Input: part model. Units: mm. Frame: model coordinates. A direction names the side the tool comes from. Give positions to 0.01 mm unless a question says otherwise; leave off trailing zeros. Loops run counter-clockwise (first coordinate to the right, second up) from the corner with the lowest first, then second, coordinate; pieces in that order, holes last. Notation, with made-up numbers: M 47.5,17.5 L 101.5,17.5 A29 ccw 101.5,45.5 Z; hole C 41.25,4.5 d8. An arc over 180 degrees is marked long. Use CSV: the item, a comma, the result in double quotes. Start each with the question number.
Q1. Pin query (flat end, axial travel): pin 1 (3.5 mm diameter, centred on x = 36, z = -3.5, fed in from +Y); pin 2 (2 mm diameter, centred on x = -11, z = -3.5, fed in from +Y); pin 3 (8 mm diameter, centred on x = 13.5, y = -80.5, fed in from -Z). Return the tip coordinate at first contact, or that it passes through.
Q2. Material intervals for line 1 along Y through (x, z) = (36.5, -1.75); line 2 along Y through (x, z) = (6.5, -5.5); line 3 along Z through (x, y) = (-1, -86.5), sorted ascending.
Q3. Section D-D, the plane y = -17. Output: boundary loops of the cut face in (x, z), plus the area to 3 significant figures.
Q4. Pull-direction query (Y, two-part tool) for faces 5 (the flat face through (-22, -88.099, -3)), 6 (the flat face through (8, -19, -5)), 7 (the cylindrical face through (-38.079, -21.806, -2.465)); classes: released by +Y, released by -Y, zero draft, split by the parting line, or undercut.
Q5. Reachability of faces 1 (the flat face through (38, -18.099, -3)), 2 (the flat face through (-36.523, -52.791, -2.535)), 3 (the flat face through (7.92, -93.59, -6.17)), 4 (the flat face through (-22, -18.099, -3)) from +Z, -Z, +X, -X, +Y, -Y: full face, straight path, thin tool, end or side. Return the list, or none.
from build123d import *

# Parameters (mm, degrees)
BOSS_EXTRUDE1_DEPTH       = 5
CHAMFER1_SIZE             = 5
BOSS_EXTRUDE2_DEPTH       = 8
CHAMFER2_SIZE2            = 5
CHAMFER2_SIZE             = 8.660254038
CHAMFER2_OF_MIRROR1_SIZE2 = 5
CHAMFER2_OF_MIRROR1_SIZE  = 8.660254038


# Some blends are built 0.0001 mm under size
with BuildPart() as part:
    # Sketch1 → Boss-Extrude1 (new body)
    # profile 1 of 2: a face of its own
    with BuildSketch(Plane.XY):
        with BuildLine():
            Line((-41.988438617, -31.098685124), (-41.988438617, -75.098685124))
            ThreePointArc((-41.988438617, -75.098685124), (-38.180826772, -84.291073279), (-28.988438617, -88.098685124))
            Line((-28.988438617, -88.098685124), (45.011561383, -88.098685124))
            ThreePointArc((45.011561383, -88.098685124), (54.203949538, -84.291073279), (58.011561383, -75.098685124))
            Line((58.011561383, -75.098685124), (58.011561383, -31.098685124))
            ThreePointArc((58.011561383, -31.098685124), (54.203949538, -21.906296968), (45.011561383, -18.098685124))
            Line((45.011561383, -18.098685124), (-28.988438617, -18.098685124))
            ThreePointArc((-28.988438617, -18.098685124), (-38.180826772, -21.906296968), (-41.988438617, -31.098685124))
        make_face()
        with BuildLine():
            ThreePointArc((-38.988438617, -75.098685124), (-36.059506429, -82.169752935), (-28.988438617, -85.098685124))
            Line((-28.988438617, -85.098685124), (45.011561383, -85.098685124))
            ThreePointArc((45.011561383, -85.098685124), (52.082629195, -82.169752935), (55.011561383, -75.098685124))
            Line((55.011561383, -75.098685124), (55.011561383, -31.098685124))
            ThreePointArc((55.011561383, -31.098685124), (52.082629195, -24.027617312), (45.011561383, -21.098685124))
            Line((45.011561383, -21.098685124), (-28.988438617, -21.098685124))
            ThreePointArc((-28.988438617, -21.098685124), (-36.059506429, -24.027617312), (-38.988438617, -31.098685124))
            Line((-38.988438617, -31.098685124), (-38.988438617, -75.098685124))
        make_face(mode=Mode.SUBTRACT)
    # profile 2 of 2: a face of its own
    with BuildSketch(Plane.XY):
        with BuildLine():
            Line((-38.988438617, -31.098685124), (-38.988438617, -75.098685124))
            ThreePointArc((-38.988438617, -75.098685124), (-36.059506429, -82.169752935), (-28.988438617, -85.098685124))
            Line((-28.988438617, -85.098685124), (45.011561383, -85.098685124))
            ThreePointArc((45.011561383, -85.098685124), (52.082629195, -82.169752935), (55.011561383, -75.098685124))
            Line((55.011561383, -75.098685124), (55.011561383, -31.098685124))
            ThreePointArc((55.011561383, -31.098685124), (52.082629195, -24.027617312), (45.011561383, -21.098685124))
            Line((45.011561383, -21.098685124), (-28.988438617, -21.098685124))
            ThreePointArc((-28.988438617, -21.098685124), (-36.059506429, -24.027617312), (-38.988438617, -31.098685124))
        make_face()
        with BuildLine():
            ThreePointArc((-33.988438617, -75.098685124), (-32.523972523, -78.63421903), (-28.988438617, -80.098685124))
            Line((-28.988438617, -80.098685124), (45.011561383, -80.098685124))
            ThreePointArc((45.011561383, -80.098685124), (48.547095289, -78.63421903), (50.011561383, -75.098685124))
            Line((50.011561383, -75.098685124), (50.011561383, -31.098685124))
            ThreePointArc((50.011561383, -31.098685124), (48.547095289, -27.563151218), (45.011561383, -26.098685124))
            Line((45.011561383, -26.098685124), (-28.988438617, -26.098685124))
            ThreePointArc((-28.988438617, -26.098685124), (-32.523972523, -27.563151218), (-33.988438617, -31.098685124))
            Line((-33.988438617, -31.098685124), (-33.988438617, -75.098685124))
        make_face(mode=Mode.SUBTRACT)
    extrude(amount=-BOSS_EXTRUDE1_DEPTH)

    # Chamfer1
    chamfer1_edges = [part.edges().sort_by_distance(p)[0] for p in [
        (8.011561383, -80.098685124, -5),
        (48.547095289, -78.63421903, -5),
        (-32.523972523, -78.63421903, -5),
        (50.011561383, -53.098685124, -5),
        (-33.988438617, -53.098685124, -5),
        (48.547095289, -27.563151218, -5),
        (-32.523972523, -27.563151218, -5),
        (8.011561383, -26.098685124, -5),
    ]]
    chamfer(chamfer1_edges, length=CHAMFER1_SIZE - 0.0001)  # a hair under: the kernel refuses the full size

    # Sketch2 → Boss-Extrude2 (add)
    with BuildSketch(Plane.XY):
        Polygon((-15.345428916, -18.098685124), (-7.774377041, -10.527633249), (23.073373404, -10.527633249), (30.644425279, -18.098685124), align=None)
    boss_extrude2 = extrude(amount=-BOSS_EXTRUDE2_DEPTH)

    # Chamfer2
    chamfer2_edges = [part.edges().sort_by_distance(p)[0] for p in [
        (7.649498182, -10.527633249, 0),
    ]]
    chamfer2_side = [part.faces().sort_by_distance(p)[0] for p in [
        (7.649498182, -10.627633249, 0),
    ]]
    chamfer(chamfer2_edges, length=CHAMFER2_SIZE, length2=CHAMFER2_SIZE2, reference=chamfer2_side[0])
    # the kernel refuses this chamfer: 8.660254038, 5 mm, written as the material it takes off along each edge
    with BuildSketch(Plane(origin=(53.049245132, -18.098685124, -8), x_dir=(0, -0.05789386240267115, 0.9983227437537926), z_dir=(-1, 0, 0))) as chamfer2_2_piece_1_section:
        with BuildLine():
            Line((5.181896449, 0), (-0.691658286, 8.935197885))
            Line((-0.691658286, 8.935197885), (-0.864572857, 8.925170374))
            ThreePointArc((-0.864572857, 8.925170374), (-0.432286429, 4.462585187), (-0.172914571, -0.010027511))
            Line((-0.172914571, -0.010027511), (0.010027511, -0.172914571))
            ThreePointArc((0.010027511, -0.172914571), (2.592291656, -0.02316616), (5.19192396, -0.172914571))
            Line((5.19192396, -0.172914571), (5.181896449, 0))
        make_face()
    chamfer2_2_piece_1 = extrude(amount=90.7994939, mode=Mode.PRIVATE)
    chamfer2_2_piece_1 = split(chamfer2_2_piece_1, bisect_by=Plane(origin=(7.649498182, -14.797310686, -5), z_dir=(0, 0, -1)), keep=Keep.TOP, mode=Mode.PRIVATE)
    add(chamfer2_2_piece_1, mode=Mode.SUBTRACT)

    # Mirror1: Boss-Extrude2 across plane
    add(boss_extrude2.mirror(Plane.ZX.offset(-53.098685124)))

    # Chamfer2 of Mirror1
    chamfer2_of_mirror1_edges = [part.edges().sort_by_distance(p)[0] for p in [
        (7.649498182, -95.669736998, 0),
    ]]
    chamfer2_of_mirror1_side = [part.faces().sort_by_distance(p)[0] for p in [
        (7.649498182, -95.569736998, 0),
    ]]
    chamfer(chamfer2_of_mirror1_edges, length=CHAMFER2_OF_MIRROR1_SIZE, length2=CHAMFER2_OF_MIRROR1_SIZE2, reference=chamfer2_of_mirror1_side[0])
    # the kernel refuses this chamfer: 8.660254038, 5 mm, written as the material it takes off along each edge
    with BuildSketch(Plane(origin=(53.049245132, -88.098685124, -8), x_dir=(0, 0.057893862402670464, 0.9983227437537926), z_dir=(-1, 0, 0))) as chamfer2_of_mirror1_2_piece_1_section:
        with BuildLine():
            Line((5.181896449, 0), (-0.691658286, -8.935197885))
            Line((-0.691658286, -8.935197885), (-0.864572857, -8.925170374))
            ThreePointArc((-0.864572857, -8.925170374), (-0.432286429, -4.462585187), (-0.172914571, 0.010027511))
            Line((-0.172914571, 0.010027511), (0.010027511, 0.172914571))
            ThreePointArc((0.010027511, 0.172914571), (2.592291656, 0.02316616), (5.19192396, 0.172914571))
            Line((5.19192396, 0.172914571), (5.181896449, 0))
        make_face()
    chamfer2_of_mirror1_2_piece_1 = extrude(amount=90.7994939, mode=Mode.PRIVATE)
    chamfer2_of_mirror1_2_piece_1 = split(chamfer2_of_mirror1_2_piece_1, bisect_by=Plane(origin=(7.649498182, -91.400059561, -5), z_dir=(0, 0, -1)), keep=Keep.TOP, mode=Mode.PRIVATE)
    add(chamfer2_of_mirror1_2_piece_1, mode=Mode.SUBTRACT)


solid = part.part
A:
1,pin 1,"y = -18.1"
1,pin 2,"y = -12.77"
1,pin 3,"z = -4.4"
2,line 1,"-88.1 to -81.85, -24.35 to -18.1"
2,line 2,"-95.67 to -92.43, -13.77 to -10.53"
2,line 3,"-5 to 0"
3,outline,"M -14.25,-5 L 29.55,-5 L 29.55,-1.26 L -14.25,-1.26 Z"
3,area,"164 mm^2"
4,face 5,"released by -Y"
4,face 6,"undercut"
4,face 7,"released by +Y"
5,face 1,"+Z, -Z, +X, +Y"
5,face 2,"-Z"
5,face 3,"-Z, +X, -X"
5,face 4,"+Z, -Z, -X, +Y"
